Input: dimensioned drawing with shaded views. Units: mm. Origin: part minimum x, y, z. A direction names the side the tool comes from. Coordinates: 2 decimals unless noted, no trailing zeros. Loops run counter-clockwise (first coordinate to the right, second up) from the corner with the lowest first, then second, coordinate; pieces in that order, holes last.
Item 1: Section query C-C, the plane y = 10.75. Return the cut outline in (x, z).
Item 2: Pin query (flat end, axial travel): pin 1 Ø1.5 at (y, z) = (5, 5) entering from -X; pin 2 Ø2 at (x, z) = (11, 2) entering from +Y; pin 3 Ø6 at (x, y) = (18, 8.5) entering from -Z; pin 4 Ø1 at (x, z) = (16, 3) entering from +Y. Return the tip coordinate at first contact, or that it passes through.
Item 3: Section query B-B, the plane z = 4. Return the cut outline in (x, y), then the cut area to 3 significant figures.
Item 4: Pull-direction query (X, two-part tool) for the marked faces 1, 2 and 3; classes: +X half, -X half, draft (parallel to the pull), parting line (faces both ways), or undercut.
Item 5: Section query D-D, the plane x = 33. Return the cut outline in (y, z).
Item 6: Line query: probe 1 along X at (y, z) = (8.5, 3.75); probe 2 along Y at (x, z) = (18, 3.5); probe 3 along X at (y, z) = (11.75, 0.75). Output: solid intervals per line, ascending.
Item 7: Section query A-A, the plane y = 8.5. Return the cut outline in (x, z).
Item 8: Reachability of the marked faces 4 and 5 from +Z, -Z, +X, -X, +Y, -Y: full face, straight path, thin tool, end or side. Return the list, or none.
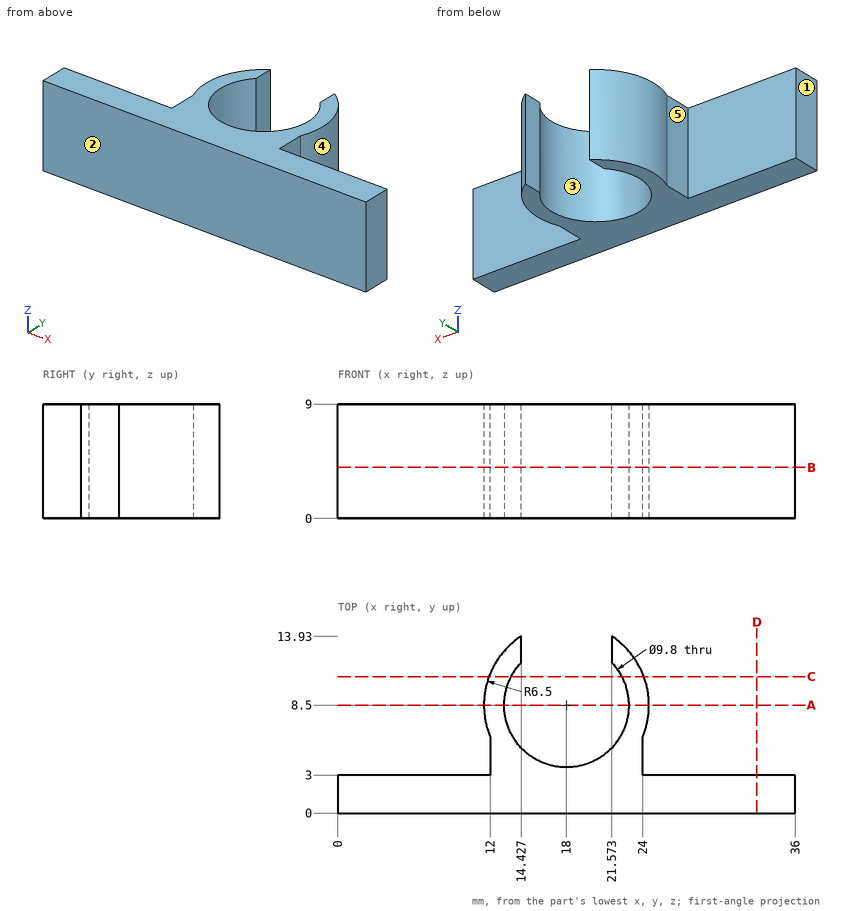
Verdict:
1. outline: (11.9, 0) - (13.65, 0) - (13.65, 9) - (11.9, 9) - close; (22.35, 0) - (24.1, 0) - (24.1, 9) - (22.35, 9) - close
2. pin 1: stops at x = 12
2. pin 2: stops at y = 11
2. pin 3: passes through
2. pin 4: stops at y = 4.29
3. outline: (0, 0) - (36, 0) - (36, 3) - (24, 3) - (24, 6) arc R6.5 ccw to (21.57, 13.93) - (21.57, 11.85) arc R4.9 cw (long way) to (14.43, 11.85) - (14.43, 13.93) arc R6.5 ccw to (12, 6) - (12, 3) - (0, 3) - close
3. area: 154 mm2
4. face 1: -X half
4. face 2: draft
4. face 3: undercut
5. outline: (0, 0) - (3, 0) - (3, 9) - (0, 9) - close
6. probe 1: x = 11.5 to 13.1, 22.9 to 24.5
6. probe 2: y = 0 to 3.6
6. probe 3: x = 12.37 to 14.33, 21.67 to 23.63
7. outline: (11.5, 0) - (13.1, 0) - (13.1, 9) - (11.5, 9) - close; (22.9, 0) - (24.5, 0) - (24.5, 9) - (22.9, 9) - close
8. face 4: +Z, -Z, +X
8. face 5: +Z, -Z, -X
